```python
from build123d import *

# Parameters (mm, degrees)
BOSS_EXTRUDE1_DEPTH = 27
CUT_EXTRUDE1_REACH  = 163.033
SKETCH2_R           = 4
CUT_EXTRUDE2_REACH  = 146.741
CUT_EXTRUDE3_START  = -26
CUT_EXTRUDE3_DEPTH  = 26


with BuildPart() as part:
    # Sketch1 → Boss-Extrude1 (new, symmetric)
    with BuildSketch(Plane.XY):
        Polygon((0, 0), (84, 0), (137.244882879, -37.282468363), (152.157870224, -15.984515211), (109.561963921, 13.841459479), (99.237588067, -0.903277318), (86.522390311, 8), (0, 8), align=None)
    extrude(amount=BOSS_EXTRUDE1_DEPTH, both=True)

    # Sketch2 → Cut-Extrude1 (cut, up to next)
    with BuildSketch(Plane(origin=(0, 8, 0), x_dir=(1, 0, 0), z_dir=(0, 1, 0)), mode=Mode.PRIVATE) as cut_extrude1_sk1:
        with Locations(Location((11, 16, 0), (0, 0, 180))):
            Circle(SKETCH2_R)
    cut_extrude1_tool1 = extrude(cut_extrude1_sk1.sketch, amount=-CUT_EXTRUDE1_REACH, mode=Mode.PRIVATE) & part.part
    # Sketch2 → Cut-Extrude1 (cut, up to next)
    with BuildSketch(Plane(origin=(0, 8, 0), x_dir=(1, 0, 0), z_dir=(0, 1, 0)), mode=Mode.PRIVATE) as cut_extrude1_sk2:
        with Locations(Location((43, 16, 0), (0, 0, 180))):
            Circle(SKETCH2_R)
    cut_extrude1_tool2 = extrude(cut_extrude1_sk2.sketch, amount=-CUT_EXTRUDE1_REACH, mode=Mode.PRIVATE) & part.part
    # Sketch2 → Cut-Extrude1 (cut, up to next)
    with BuildSketch(Plane(origin=(0, 8, 0), x_dir=(1, 0, 0), z_dir=(0, 1, 0)), mode=Mode.PRIVATE) as cut_extrude1_sk3:
        with Locations(Location((75, 16, 0), (0, 0, 180))):
            Circle(SKETCH2_R)
    cut_extrude1_tool3 = extrude(cut_extrude1_sk3.sketch, amount=-CUT_EXTRUDE1_REACH, mode=Mode.PRIVATE) & part.part
    # Sketch2 → Cut-Extrude1 (cut, up to next)
    with BuildSketch(Plane(origin=(0, 8, 0), x_dir=(1, 0, 0), z_dir=(0, 1, 0)), mode=Mode.PRIVATE) as cut_extrude1_sk4:
        with Locations(Location((43, -16, 0), (0, 0, 180))):
            Circle(SKETCH2_R)
    cut_extrude1_tool4 = extrude(cut_extrude1_sk4.sketch, amount=-CUT_EXTRUDE1_REACH, mode=Mode.PRIVATE) & part.part
    # Sketch2 → Cut-Extrude1 (cut, up to next)
    with BuildSketch(Plane(origin=(0, 8, 0), x_dir=(1, 0, 0), z_dir=(0, 1, 0)), mode=Mode.PRIVATE) as cut_extrude1_sk5:
        with Locations(Location((75, -16, 0), (0, 0, 180))):
            Circle(SKETCH2_R)
    cut_extrude1_tool5 = extrude(cut_extrude1_sk5.sketch, amount=-CUT_EXTRUDE1_REACH, mode=Mode.PRIVATE) & part.part
    # Sketch2 → Cut-Extrude1 (cut, up to next)
    with BuildSketch(Plane(origin=(0, 8, 0), x_dir=(1, 0, 0), z_dir=(0, 1, 0)), mode=Mode.PRIVATE) as cut_extrude1_sk6:
        with Locations(Location((11, -16, 0), (0, 0, 180))):
            Circle(SKETCH2_R)
    cut_extrude1_tool6 = extrude(cut_extrude1_sk6.sketch, amount=-CUT_EXTRUDE1_REACH, mode=Mode.PRIVATE) & part.part
    add(cut_extrude1_tool1.solids().sort_by_distance((11, 8, -16))[0], mode=Mode.SUBTRACT)
    add(cut_extrude1_tool2.solids().sort_by_distance((43, 8, -16))[0], mode=Mode.SUBTRACT)
    add(cut_extrude1_tool3.solids().sort_by_distance((75, 8, -16))[0], mode=Mode.SUBTRACT)
    add(cut_extrude1_tool4.solids().sort_by_distance((43, 8, 16))[0], mode=Mode.SUBTRACT)
    add(cut_extrude1_tool5.solids().sort_by_distance((75, 8, 16))[0], mode=Mode.SUBTRACT)
    add(cut_extrude1_tool6.solids().sort_by_distance((11, 8, 16))[0], mode=Mode.SUBTRACT)

    # Sketch3 → Cut-Extrude2 (cut, up to next)
    with BuildSketch(Plane(origin=(109.609728898, -76.749558436, 0), x_dir=(0, 0, -1), z_dir=(0.819152044288994, -0.5735764363510429, 0)), mode=Mode.PRIVATE) as cut_extrude2_sk1:
        Polygon((-5, 74.180420653), (5, 74.180420653), (5, 64.180420653), (17.5, 64.180420653), (17.5, 56.180420653), (-17.5, 56.180420653), (-17.5, 64.180420653), (-5, 64.180420653), align=None)
    cut_extrude2_tool1 = extrude(cut_extrude2_sk1.sketch, amount=-CUT_EXTRUDE2_REACH, mode=Mode.PRIVATE) & part.part
    add(cut_extrude2_tool1.solids().sort_by_distance((145.486271, -25.512547, 0))[0], mode=Mode.SUBTRACT)

    # Sketch5 → Cut-Extrude3 (cut)
    with BuildSketch(Plane(origin=(42.548141325, 60.765043225, 0), x_dir=(0.8191520442889936, -0.5735764363510437, 0), z_dir=(0.5735764363510436, 0.8191520442889935, 0)).offset(CUT_EXTRUDE3_START)):
        with BuildLine():
            Line((126.249743807, 27), (150.866337787, 27))
            Line((150.866337787, 27), (150.866337787, -27))
            Line((150.866337787, -27), (126.249743807, -27))
            ThreePointArc((126.249743807, -27), (133.80877172, 0), (126.249743807, 27))
        make_face()
    extrude(amount=CUT_EXTRUDE3_DEPTH, mode=Mode.SUBTRACT)


solid = part.part
```
Build history of the part. All positions in model axes, mm. A direction names the side the tool comes from. Coordinates: 2 decimals unless noted, no trailing zeros. Order: outer loops, then holes, each group sorted by start corner. A loop starts at its lowest first (then second) coordinate and runs counter-clockwise, first axis right, second up. Notation, with made-up numbers: M -0.75,6.5 L 51.25,6.5 A15 cw 51.25,21.5 Z; hole C 59.5,59 d7. An arc over 180 degrees is marked long. One line per question, with ' | ' between items. Start each with the question number.
1. Cut at B-B (y = 2.5). Count the separate pieces of the cut face and the enclosed holes in it, plus the area to 3 significant figures.
2. Wall check: line 1 along Z through (x, y) = (11, 4); line 2 along Z through (x, y) = (107.5, 10); line 3 along Y through (x, z) = (16, -21.5). Give the ranges that are in metal, low to high. Write a range as [from, to].
3. Cut at A-A (x = 75). Write the cut outline in (y, z).
4. Cut at D-D (z = 7). Write the cut outline in (x, y).
5. Flat gauge pins, fed straight in: P1, Ø6, axis at y = -6.5, z = -3.5, coming from the +X side; P2, Ø12, axis at y = -16, z = -2, coming from the +X side; P3, Ø13, axis at x = 75, z = 16, coming from the +Y side; P4, Ø12, axis at y = -32, z = -18.5, coming from the +X side. Where does each tip first touch, or does it go through?
6. Cut at C-C (z = -14). Write the cut outline in (x, y), plus the area to 3 significant figures.
7. Mould opens along Z. For faces 5 (the face through (128, -5, 5)), 6 (the face through (89, -1, 27)), 7 (the face through (105.62, 8.21, 18.6)), 8 (the face through (11.521, 4.056, 19.966)) say: +Z half, -Z half, draft (parallel to the pull), parting line (faces both ways), or undercut.
8. Tool access for faces 1 (the face through (125.32, -9.4, -11.16)), 2 (the face through (44, 8, 0)), 3 (the face through (128, -5, -5)), 4 (the face through (105.62, 8.21, -18.29)): list every direction of +Z, -Z, +X, -X, +Y, -Y with a clear straight run to the whole face (end or side of a thin tool).
The answers:
1) separate pieces: 3 | enclosed holes: 6 | area: 5,690 mm2
2) line 1: z = [-27, -20], [-12, 12], [20, 27] | line 2: z = [-27, -5], [5, 27] | line 3: y = [0, 8]
3) outline: M 0,-27 L 8,-27 L 8,-20 L 0,-20 Z; M 0,-12 L 8,-12 L 8,12 L 0,12 Z; M 0,20 L 8,20 L 8,27 L 0,27 Z
4) outline: M 0,0 L 84,0 L 136.86,-37.01 L 141.45,-30.46 L 86.52,8 L 0,8 Z; M 103.83,5.65 L 146.03,-23.9 L 151.77,-15.71 L 109.56,13.84 Z
5) P1: stops at x = 142.32 | P2: stops at x = 151.96 | P3: stops at y = 8 | P4: stops at x = 141.38
6) outline: M 0,0 L 7.54,0 L 7.54,8 L 0,8 Z; M 14.46,0 L 39.54,0 L 39.54,8 L 14.46,8 Z; M 46.46,0 L 71.54,0 L 71.54,8 L 46.46,8 Z; M 78.46,0 L 84,0 L 135.67,-36.18 L 140.26,-29.63 L 86.52,8 L 78.46,8 Z; M 103.83,5.65 L 144.85,-23.07 L 150.59,-14.88 L 109.56,13.84 Z | area: 1,530 mm2
7) face 5: undercut | face 6: +Z half | face 7: draft | face 8: undercut
8) face 1: none | face 2: +Z, -Z, -X, +Y | face 3: +X, +Y | face 4: +Z, -Z, +Y
